The listing builds one solid part. Answer for the finished solid, in the listing's coordinates (mm). A direction names the side the tool comes from. Give positions to 0.01 mm unless a question says otherwise; leave off trailing zeros. Loops run counter-clockwise (first coordinate to the right, second up) from the corner with the lowest first, then second, coordinate; pieces in that order, holes last. Notation, with made-up numbers: M -35.75,10 L -31.75,10 A19 cw -31.75,15 Z; hole C 78,-4.75 d2. An arc over 180 degrees is marked long. One line per item, written item: value. Start each with the question number.
Q1. Consider L1, parallel to Z at x = 0, y = 25.5; L2, parallel to X at y = 16, z = 0; L3, parallel to Z at x = 2.5, y = 28.5. Determine where each line is inside the solid, lowest interval first.
Q2. A cutting plane is placed at B-B, the plane z = -6. Determine the outline of the cut face in (x, y).
Q3. Flat-ended cylindrical pins translate along their axes: pin 1 (5 mm diameter, centred on y = 19, z = 7.5, fed in from +X); pin 2 (2 mm diameter, centred on x = -6, y = 19, fed in from +Z); pin 3 (12 mm diameter, centred on y = 16, z = -7.5, fed in from +X). Find the tip coordinate at first contact, or state that the pin passes through.
Q4. A cutting plane is placed at A-A, the plane y = 22.25. Determine the outline of the cut face in (x, z), and give its area (3 significant figures).
Q5. The mould has two halves that part along Z. Classify faces 1 (the flat face through (4.3, 0, 4.3)), 2 (the cylindrical face through (2.98, 25.56, 4.68)): +Z half, -Z half, draft (parallel to the pull), parting line (faces both ways), or undercut.
Q6. For faces 3 (the flat face through (-4, 21, -2)), 4 (the flat face through (-4, 9, -2)), 5 (the flat face through (4.3, 30, 4.3)), determine the directions among +Z, -Z, +X, -X, +Y, -Y from which every point of the face is accessible in a straight line to the end or side of a thin tool.
Q7. A cutting plane is placed at C-C, the plane x = -5. Determine the outline of the cut face in (y, z).
Q8. A cutting plane is placed at D-D, the plane y = 14.5. Determine the outline of the cut face in (x, z), and give its area (3 significant figures).
from build123d import *

# Parameters (mm, degrees)
SKETCH1_R           = 10
BOSS_EXTRUDE1_DEPTH = 15
SKETCH2_R           = 5.55
CUT_EXTRUDE1_DEPTH  = 9


with BuildPart() as part:
    # Sketch1 → Boss-Extrude1 (new body)
    with BuildSketch(Plane(origin=(0, 0, 0), x_dir=(1, 0, 0), z_dir=(0, 1, 0))):
        Circle(SKETCH1_R)
    boss_extrude1 = extrude(amount=BOSS_EXTRUDE1_DEPTH)

    # Sketch2 → Cut-Extrude1 (cut)
    with BuildSketch(Plane.XZ):
        Circle(SKETCH2_R)
    cut_extrude1 = extrude(amount=-CUT_EXTRUDE1_DEPTH, mode=Mode.SUBTRACT)

    # Sketch3 → Cut-Revolve3 (revolve, cut)
    with BuildSketch(Plane.XY):
        with BuildLine():
            Line((-4.241288088, 9), (0, 9))
            Line((0, 9), (0, 15))
            Line((0, 15), (-2.25, 15))
            ThreePointArc((-2.25, 15), (-2.295576741, 14.479055467), (-2.430922138, 13.97393957))
            Line((-2.430922138, 13.97393957), (-4.241288088, 9))
        make_face()
    cut_revolve3 = revolve(axis=Axis((0, 15, 0), (0, 1, 0)), mode=Mode.SUBTRACT)

    # Mirror1: Boss-Extrude1, Cut-Extrude1, Cut-Revolve3 across plane
    add(boss_extrude1.mirror(Plane.ZX.offset(15)))
    add(cut_extrude1.mirror(Plane.ZX.offset(15)), mode=Mode.SUBTRACT)
    add(cut_revolve3.mirror(Plane.ZX.offset(15)), mode=Mode.SUBTRACT)


solid = part.part
Answer block:
1. L1: -10 to -5.55, 5.55 to 10
1. L2: -10 to -2.42, 2.42 to 10
1. L3: -9.68 to -4.96, 4.96 to 9.68
2. outline: M -8,0 L 8,0 L 8,30 L -8,30 Z
3. pin 1: x = 8.66
3. pin 2: z = 8.66
3. pin 3: x = 9.89
4. outline: C 0,0 d20; hole C 0,0 d11.1
4. area: 217 mm^2
5. face 1: draft
5. face 2: undercut
6. face 3: +Y
6. face 4: -Y
6. face 5: +Z, -Z, +X, -X, +Y
7. outline: M 0,-8.66 L 30,-8.66 L 30,-2.41 L 21,-2.41 L 21,2.41 L 30,2.41 L 30,8.66 L 0,8.66 L 0,2.41 L 9,2.41 L 9,-2.41 L 0,-2.41 Z
8. outline: C 0,0 d20; hole C 0,0 d4.58
8. area: 298 mm^2
